Answer from the drawing. Dimensions are ordinates in mm from the lowest x, y and z of the part. A direction names the side the tool comes from. Round coordinates to 2 decimals unless told otherwise and drop trailing zeros. Loops run counter-clockwise (first coordinate to the right, second up) from the corner with the lowest first, then second, coordinate; pieces in that order, holes last. Notation, with made-up numbers: (15.25, 44.25) -> (54.25, 44.25) arc R16 ccw to (54.25, 50.25) -> close; hole circle Ø1 at (74.5, 86.5). An arc over 180 degrees is marked (long way). One line per question, with ' | ' between items.
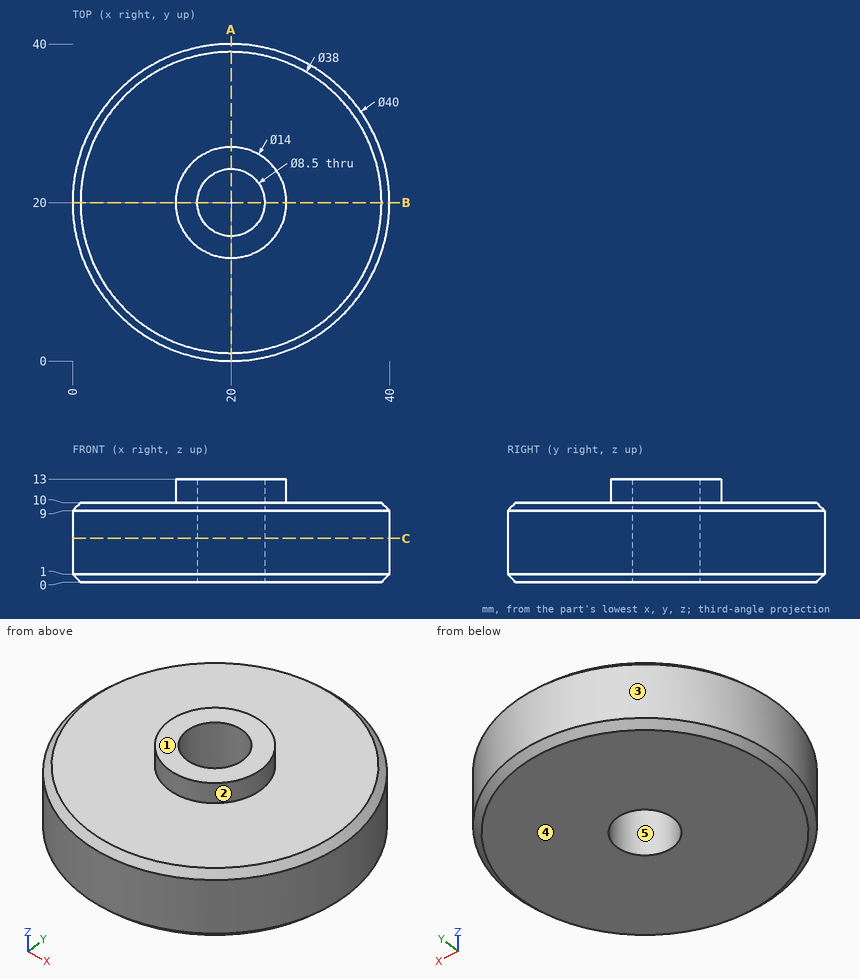
Q1. For a pull along X with two mould halves and no side action, classify the marked faces 3, 4 and 5 as pulls with the +X half, pulls with the -X half, needs draft (parallel to the pull), parting line crosses it, or undercut.
Numbers:
face 3: parting line crosses it | face 4: needs draft | face 5: undercut
Q2. For the marked faces 1 and 2, determine the directions among +Z, -Z, +X, -X, +Y, -Y from which every point of the face is accessible in a straight line to the end or side of a thin tool.
Numbers:
face 1: +Z, +X, -X, +Y, -Y | face 2: +Z
Q3. Given pin 1 Ø4 at (y, z) = (9.5, 9) entering from -X; pin 2 Ø5 at (x, z) = (25.5, 6) entering from +Y; pin 3 Ø3 at (y, z) = (31.5, 10.5) entering from -X, each flat-ended and moving along its own axis, determine where each tip first touches the part or whether it passes through.
Numbers:
pin 1: x = 1.9 | pin 2: y = 39.77 | pin 3: x = 3.37
Q4. A cutting plane is placed at C-C on z = 5.5. Give the vertices of the cut face in (x, y), plus the area to 3 significant figures.
Numbers:
outline: circle Ø40 at (20, 20); hole circle Ø8.5 at (20, 20) | area: 1,200 mm^2
Q5. A cutting plane is placed at A-A on x = 20. Give the vertices of the cut face in (y, z).
Numbers:
outline: (0, 1) -> (1, 0) -> (15.75, 0) -> (15.75, 13) -> (13, 13) -> (13, 10) -> (1, 10) -> (0, 9) -> close; (24.25, 0) -> (39, 0) -> (40, 1) -> (40, 9) -> (39, 10) -> (27, 10) -> (27, 13) -> (24.25, 13) -> close
Q6. Find the intervals of material crossed by line 1 (Y direction, x = 20, z = 10.25); line 2 (Y direction, x = 20, z = 8.5); line 3 (Z direction, x = 24, y = 11), in increasing order. Write a range as from..to.
Numbers:
line 1: 13..15.75, 24.25..27 | line 2: 0..15.75, 24.25..40 | line 3: 0..10
